The listing builds one solid part. Answer for the finished solid, in the listing's coordinates (mm). Face numbers are marked on the shaded views. A direction names the side the tool comes from. Coordinates: 2 decimals unless noted, no trailing zeros. Loops run counter-clockwise (first coordinate to the right, second up) from the corner with the lowest first, then second, coordinate; pieces in that order, holes last. Notation, with made-up numbers: (61, 38.25) - (114, 38.25) arc R14 cw to (114, 56.25) - close; hole circle Ø5 at (34.25, 52). An arc over 180 degrees is marked (long way). One line per question, with ' | ' between items.
from build123d import *

# Parameters (mm, degrees)
SKETCH_2_W          = 62
SKETCH_2_H          = 82
EXTRUDE_2_DEPTH     = 30
SKETCH_3_R          = 12
CUT_EXTRUDE_1_DEPTH = 60.514704065
CUT_EXTRUDE_2_DEPTH = 60.514704065
HOLE_WIZARD_M4_1_D  = 3.3
HOLE_WIZARD_M4_2_D  = 3.3


with BuildPart() as part:
    # 草图2 → 凸台-拉伸2 (new body)
    with BuildSketch(Plane(origin=(0, 0, 0), x_dir=(0, 0, -1), z_dir=(1, 0, 0))):
        Rectangle(SKETCH_2_W, SKETCH_2_H)
    extrude(amount=EXTRUDE_2_DEPTH)

    # 草图3 → 切除-拉伸1 (cut, through all)
    with BuildSketch(Plane.ZY):
        with Locations((0, 20)):
            Circle(SKETCH_3_R)
    extrude(amount=-CUT_EXTRUDE_1_DEPTH, mode=Mode.SUBTRACT)

    # 草图7 → 切除-拉伸2 (cut, through all)
    with BuildSketch(Plane(origin=(30, 0, 0), x_dir=(0, 0, -1), z_dir=(1, 0, 0))):
        Polygon((-31, 29), (-21, 29), (-21, 4), (21, 4), (21, 29), (31, 29), (31, -41), (-31, -41), align=None)
    extrude(amount=-CUT_EXTRUDE_2_DEPTH, mode=Mode.SUBTRACT)

    # M4 螺纹孔1 (through all)
    with Locations(Plane.ZY):
        with Locations((-11.313708499, 31.313708499), (11.313708499, 8.686291501), (11.313708499, 31.313708499), (16, 20), (-11.313708499, 8.686291501), (-16, 20)):
            Hole(HOLE_WIZARD_M4_1_D / 2)

    # M4 螺纹孔2 (through all)
    with Locations(Plane(origin=(0, 29, 0), x_dir=(-1, 0, 0), z_dir=(0, -1, 0))):
        with Locations((-6, 26), (-24, 26), (-6, -26), (-24, -26)):
            Hole(HOLE_WIZARD_M4_2_D / 2)


solid = part.part
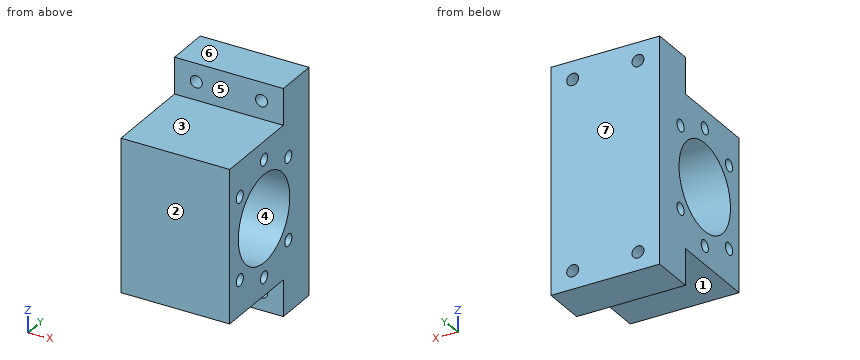
Item 1: Find section A-A, the plane y = 20. Write down the section's boundary in (x, z).
Taken from the geometry:
outline: (0, -21) - (30, -21) - (30, -17.65) - (0, -17.65) - close; (0, -14.35) - (30, -14.35) - (30, -12) - (0, -12) - close; (0, 12) - (30, 12) - (30, 14.35) - (0, 14.35) - close; (0, 17.65) - (30, 17.65) - (30, 21) - (0, 21) - close
Item 2: The mould has two halves that part along Y. Classify the marked faces 4, 5, 6 and 7: pulls with the +Y half, pulls with the -Y half, needs draft (parallel to the pull), parting line crosses it, or undercut.
Taken from the geometry:
face 4: undercut | face 5: pulls with the -Y half | face 6: needs draft | face 7: pulls with the +Y half
Item 3: Each of these flat-tipped pins is pushed along its axis until it touches: pin 1 Ø12 at (x, y) = (8.5, 20) entering from +Z; pin 2 Ø4 at (x, z) = (6, -26) entering from -Y; pin 3 Ø3 at (y, z) = (31.31, -11.31) entering from +X; pin 4 Ø7.5 at (x, y) = (16, 14) entering from -Z. Where does it stop, or does it pass through?
Taken from the geometry:
pin 1: stops at z = 21 | pin 2: stops at y = 29 | pin 3: passes through | pin 4: stops at z = -21
Item 4: Find the intervals of material crossed by line 1 (X direction, y = 33.25, z = -26); line 2 (Z direction, x = 24, y = 34.5); line 3 (Z direction, x = 6.5, y = 30), in increasing order. Write a range as [from, to].
Taken from the geometry:
line 1: x = [0, 4.35], [7.65, 22.35], [25.65, 30] | line 2: z = [-31, -27.65], [-24.35, 24.35], [27.65, 31] | line 3: z = [-31, -27.57], [-24.43, -12.31], [-10.32, -6.63], [6.63, 10.32], [12.31, 24.43], [27.57, 31]
Item 5: Find section D-D, the plane y = 36. Write down the section's boundary in (x, z), plus the area to 3 significant figures.
Taken from the geometry:
outline: (0, -31) - (30, -31) - (30, 31) - (0, 31) - close; hole circle Ø3.3 at (6, -26); hole circle Ø3.3 at (6, 26); hole circle Ø3.3 at (24, -26); hole circle Ø3.3 at (24, 26) | area: 1,830 mm2
Item 6: Which of the six approach directions +Z, -Z, +X, -X, +Y, -Y give full straight-line access (tool end or side, diameter ignored) to the marked faces 1, 2 and 3?
Taken from the geometry:
face 1: -Z, +X, -X, -Y | face 2: +Z, -Z, +X, -X, -Y | face 3: +Z, +X, -X, -Y
Item 7: Find section B-B, the plane z = 16. Write down the section's boundary in (x, y), plus the area to 3 significant figures.
Taken from the geometry:
outline: (0, 4) - (30, 4) - (30, 18.35) - (0, 18.35) - close; (0, 21.65) - (30, 21.65) - (30, 41) - (0, 41) - close | area: 1,010 mm2
Item 8: Find section C-C, the plane z = 26. Write down the section's boundary in (x, y).
Taken from the geometry:
outline: (0, 29) - (4.35, 29) - (4.35, 41) - (0, 41) - close; (7.65, 29) - (22.35, 29) - (22.35, 41) - (7.65, 41) - close; (25.65, 29) - (30, 29) - (30, 41) - (25.65, 41) - close
